Job drawing, mm, ordinate dimensions from the low corner. One solid piece. Round coordinates to 2 decimals unless told otherwise and drop trailing zeros. Write each loop counter-clockwise with the first axis right and the second up, starting at its lowest first coordinate (ties: lowest second). Pieces come first, ordered by that corner, then holes.
1) Saw through at C-C (y = 18). Write the cut outline in (x, z).
2) Flat gauge pins, fed straight in: pin 1 (3.5 mm diameter, centred on x = 47.5, z = 9, fed in from -Y); pin 2 (5 mm diameter, centred on y = 38, z = 7, fed in from -X); pin 3 (1.5 mm diameter, centred on x = 60, z = 8, fed in from +Y); pin 4 (10 mm diameter, centred on x = 14, y = 46.5, fed in from +Z). Where does each tip first touch, or does it go through?
3) Saw through at A-A (x = 18). Write the cut outline in (y, z), plus the area to 3 significant figures.
4) Wall check: probe 1 along Y at (x, z) = (18, 4.5); probe 2 along X at (y, z) = (18, 8.75); probe 3 along Z at (x, y) = (58, 7). Give the ranges that are in metal, low to high.
5) Saw through at B-B (z = 4.5). Write the cut outline in (x, y).
6) Saw through at D-D (x = 50.5). Write the cut outline in (y, z).
7) Pull direction X, two halves, no side cores. Call the marked faces 1, 2 and 3: +X half, -X half, draft (parallel to the pull), parting line (faces both ways), or undercut.
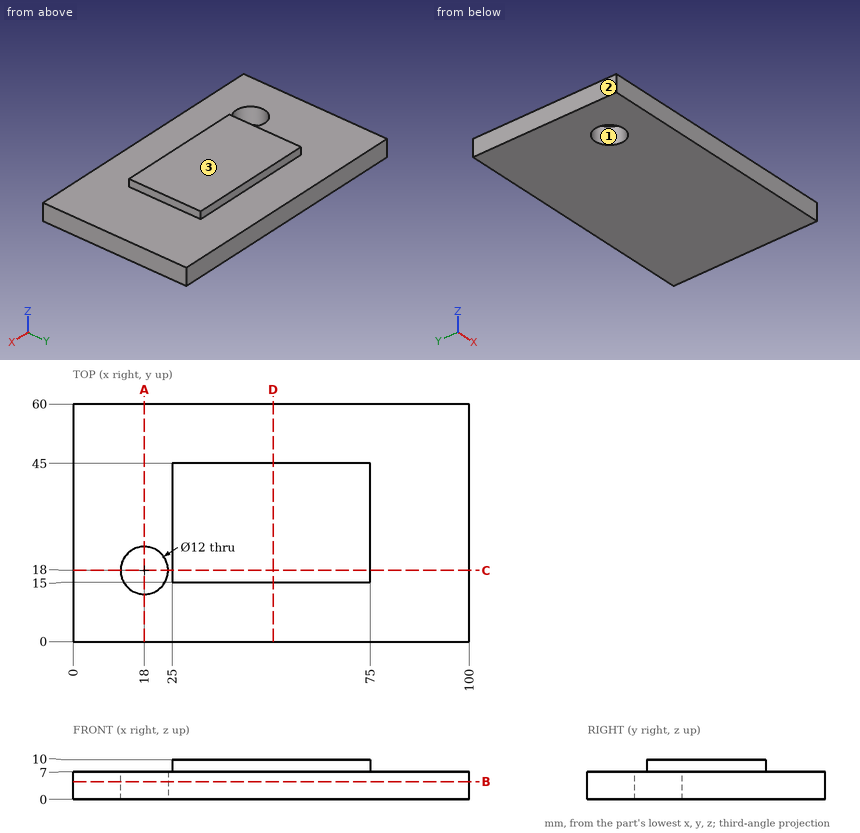
Evaluation:
1. outline: (0, 0) - (12, 0) - (12, 7) - (0, 7) - close; (24, 0) - (100, 0) - (100, 7) - (75, 7) - (75, 10) - (25, 10) - (25, 7) - (24, 7) - close
2. pin 1: stops at y = 15
2. pin 2: stops at x = 0
2. pin 3: stops at y = 45
2. pin 4: stops at z = 7
3. outline: (0, 0) - (12, 0) - (12, 7) - (0, 7) - close; (24, 0) - (60, 0) - (60, 7) - (24, 7) - close
3. area: 336 mm2
4. probe 1: y = 0 to 12, 24 to 60
4. probe 2: x = 25 to 75
4. probe 3: z = 0 to 7
5. outline: (0, 0) - (100, 0) - (100, 60) - (0, 60) - close; hole circle Ø12 at (18, 18)
6. outline: (0, 0) - (60, 0) - (60, 7) - (45, 7) - (45, 10) - (15, 10) - (15, 7) - (0, 7) - close
7. face 1: undercut
7. face 2: -X half
7. face 3: draft
